Model file for the job. Use its own axes, mm. A direction names the side the tool comes from. Coordinates: 2 decimals unless noted, no trailing zeros. Write each loop counter-clockwise with the first axis right and the second up, starting at its lowest first coordinate (ties: lowest second). Pieces come first, ordered by that corner, then holes. Notation, with made-up numbers: (10, 30.5) -> (66, 30.5) arc R16 cw to (66, 57.5) -> close; hole circle Ø1 at (-20.75, 9). An arc over 180 degrees is marked (long way). Answer as a JSON object with one key per item and string values. Group by question number.
from build123d import *

# Parameters (mm, degrees)
BOSS_EXTRUDE3_DEPTH                      = 50.8
BOSS_EXTRUDE4_DEPTH                      = 58.906461925
MIRROR1_AT_THE_SECOND_PLANE_COPY_1_DEPTH = 58.906461925


with BuildPart() as part:
    # Sketch3 → Boss-Extrude3 (new body)
    with BuildSketch(Plane.XY):
        Polygon((0, 0), (14.568841483, -20.806461925), (471.768841483, -20.806461925), (486.337682967, 0), (459.659775761, 38.1), (26.677907206, 38.1), align=None)
    extrude(amount=BOSS_EXTRUDE3_DEPTH)

    # Sketch4 → Boss-Extrude4 (add)
    with BuildSketch(Plane(origin=(0, 38.1, 0), x_dir=(1, 0, 0), z_dir=(0, 1, 0))):
        with BuildLine():
            Line((45.727907206, -55.5625), (45.727907206, -50.8))
            Line((45.727907206, -50.8), (58.427907206, -50.8))
            Line((58.427907206, -50.8), (58.427907206, -55.5625))
            ThreePointArc((58.427907206, -55.5625), (52.077907206, -61.9125), (45.727907206, -55.5625))
        make_face()
    boss_extrude4 = extrude(amount=-BOSS_EXTRUDE4_DEPTH)

    # Mirror1: Boss-Extrude4 across plane
    add(boss_extrude4.mirror(Plane(origin=(243.205, 0, 0), x_dir=(0, 0, 1), z_dir=(1, 0, 0))))

    # Mirror1 at the second plane: Boss-Extrude4 across plane
    add(boss_extrude4.mirror(Plane.XY.offset(25.4)))

    # Mirror1 at the second plane copy 1 sketc → Mirror1 at the second plane copy 1 (add)
    with BuildSketch(Plane(origin=(486.41, 38.1, 50.8), x_dir=(-1, 0, 0), z_dir=(0, 1, 0))):
        with BuildLine():
            Line((45.727907206, -55.5625), (45.727907206, -50.8))
            Line((45.727907206, -50.8), (58.427907206, -50.8))
            Line((58.427907206, -50.8), (58.427907206, -55.5625))
            ThreePointArc((58.427907206, -55.5625), (52.077907206, -61.9125), (45.727907206, -55.5625))
        make_face()
    extrude(amount=-MIRROR1_AT_THE_SECOND_PLANE_COPY_1_DEPTH)


solid = part.part
(1) Cut at B-B on y = 6. List the corners of the cut face in (x, z).
(2) Cut at C-C on x = 399. List the corners of the cut face in (y, z).
(3) Pull direction X, two halves, no side cores. Call faces 1 (the face through (478.95, -10.55, 25.04)), 2 (the face through (28, 9, 50.8)), 3 (the face through (241, 9, 50.8)): released by +X, released by -X, zero draft, split by the parting line, or undercut.
(4) Wall check: probe 1 along Z at (x, y) = (262.5, 15.5); probe 2 along X at (y, z) = (11, 12); probe 3 along X at (y, z) = (-3.5, 19.5). Give the ranges that are in metal, low to high.
(5) Cut at D-D on y = 29.5. List the corners of the cut face in (x, z), plus the area to 3 significant figures.
(6) Cut at A-A on z = 20.5. List the corners of the cut face in (x, y), plus the area to 3 significant figures.
(7) 3-axis set-ups, long thin cutter, end or side, ignore diameter. For faces 4 (the face through (28, 9, 0)), 5 (the face through (458, 9, 50.8)), 6 (the face through (458, 9, 0)): which of +Z, -Z, +X, -X, +Y, -Y reach the whole face in a straight line?
(8) Pin check, flat tips, straight feed: pin 1 (2 mm diameter, centred on x = 330, y = 11.5, fed in from +Z); pin 2 (1.4 mm diameter, centred on y = 13.5, z = -3, fed in from +X); pin 3 (1.4 mm diameter, centred on y = -4.5, z = -1.5, fed in from -X). Stop position of each tip, or through.
Results found:
{
 "1": {"outline": "(4.2, 0) -> (45.73, 0) -> (45.73, -4.76) arc R6.35 ccw to (58.43, -4.76) -> (58.43, 0) -> (427.98, 0) -> (427.98, -4.76) arc R6.35 ccw to (440.68, -4.76) -> (440.68, 0) -> (482.14, 0) -> (482.14, 50.8) -> (440.68, 50.8) -> (440.68, 55.56) arc R6.35 ccw to (427.98, 55.56) -> (427.98, 50.8) -> (58.43, 50.8) -> (58.43, 55.56) arc R6.35 ccw to (45.73, 55.56) -> (45.73, 50.8) -> (4.2, 50.8) -> close"},
 "2": {"outline": "(-20.81, 0) -> (38.1, 0) -> (38.1, 50.8) -> (-20.81, 50.8) -> close"},
 "3": {"face 1": "released by +X", "face 2": "zero draft", "face 3": "undercut"},
 "4": {"probe 1": "z = 0 to 50.8", "probe 2": "x = 7.7 to 478.64", "probe 3": "x = 2.45 to 483.89"},
 "5": {"outline": "(20.66, 0) -> (45.73, 0) -> (45.73, -4.76) arc R6.35 ccw to (58.43, -4.76) -> (58.43, 0) -> (427.98, 0) -> (427.98, -4.76) arc R6.35 ccw to (440.68, -4.76) -> (440.68, 0) -> (465.68, 0) -> (465.68, 50.8) -> (440.68, 50.8) -> (440.68, 55.56) arc R6.35 ccw to (427.98, 55.56) -> (427.98, 50.8) -> (58.43, 50.8) -> (58.43, 55.56) arc R6.35 ccw to (45.73, 55.56) -> (45.73, 50.8) -> (20.66, 50.8) -> close", "area": "23,100 mm²"},
 "6": {"outline": "(0, 0) -> (14.57, -20.81) -> (471.77, -20.81) -> (486.34, 0) -> (459.66, 38.1) -> (26.68, 38.1) -> close", "area": "27,300 mm²"},
 "7": {"face 4": "-Z, -X, +Y, -Y", "face 5": "+Z, +X, +Y, -Y", "face 6": "-Z, +X, +Y, -Y"},
 "8": {"pin 1": "stops at z = 50.8", "pin 2": "stops at x = 440.68", "pin 3": "stops at x = 45.73"}
}
